Geometry check sheet. Reference: the model listing, model coordinates, mm. Face numbers are marked on the shaded views. A direction names the side the tool comes from. Give positions to 0.01 mm unless a question says otherwise; leave off trailing zeros. Write each loop counter-clockwise with the first axis right and the second up, starting at its lowest first coordinate (ties: lowest second). Pieces come first, ordered by that corner, then holes.
(1) Depth check by flat-ended pin: P1, Ø13, axis at x = 10, z = 35.5, coming from the -Y side; P2, Ø3, axis at y = 114.5, z = 40, coming from the -X side; P3, Ø12, axis at x = 17, y = 60.5, coming from the -Z side; P4, Ø13, axis at x = 16, z = 33.5, coming from the -Y side. Enter the tip coordinate at first touch or a pass-through.
(2) Thickness scan on line 1 along Z through (x, y) = (3, 41); line 2 along Y through (x, z) = (19, 22.86); line 3 along Z through (x, y) = (8.5, 0). Record the ranges inside material, lowest first.
(3) Cross-section at B-B (x = 12.7). Count the separate pieces of the cut face and the enclosed holes in it, and give its area (3 significant figures).
(4) Cross-section at A-A (y = 215.9). Record the boundary of the cut face in (x, z).
(5) Tool access check on the marked faces 5, 6 and 7. Record the directions out of +Z, -Z, +X, -X, +Y, -Y that give a thin tool (end or side, any length) a straight path to the whole face; none if there is none.
(6) Mould release check, pull along Z, two halves, no side actions. Record for the marked faces 1, 2, 3 and 4: +Z half, -Z half, draft (parallel to the pull), parting line (faces both ways), or undercut.
```python
from build123d import *

# Parameters (mm, degrees)
SKETCH3_W               = 50.8
SKETCH3_H               = 254
BOSS_EXTRUDE1_DEPTH     = 25.4
SKETCH4_R               = 4.7117
CUT_EXTRUDE1_DEPTH      = 246.225128402
SKETCH5_R               = 2.413
CUT_EXTRUDE2_DEPTH      = 246.225128402
SKETCH6_W               = 45.72
SKETCH6_H               = 85.725
CUT_EXTRUDE3_DEPTH      = 246.225128402
SKETCH7_W               = 15.24
SKETCH7_H               = 85.725
CUT_EXTRUDE4_DEPTH      = 1.4986
SKETCH8_W               = 15.24
SKETCH8_H               = 85.725
CUT_EXTRUDE5_DEPTH      = 1.4986
SKETCH9_W               = 30.48
SKETCH9_H               = 230.759
CUT_EXTRUDE6_DEPTH      = 246.225128402
FILLET5_R               = 6.35
SKETCH14_W              = 25.4
SKETCH14_H              = 254
BOSS_EXTRUDE2_DEPTH     = 12.7
FILLET8_R               = 38.1
FILLET9_R               = 9.525
FILLET10_R              = 10.16
FILLET11_R              = 15.24
FILLET12_R              = 5.08
SKETCH18_R              = 2.413
CUT_EXTRUDE8_DEPTH      = 251.804904258
CUT_EXTRUDE9_DEPTH      = 248.386090151
FILLET13_R              = 3.175
SKETCH20_R              = 6.35
CUT_EXTRUDE10_DEPTH     = 248.386090151
CUT_EXTRUDE11_START     = -254
CUT_EXTRUDE11_OUTLINE_W = 1.4986
CUT_EXTRUDE11_OUTLINE_H = 63.5
CUT_EXTRUDE11_DEPTH     = 254


# Read off the part's stored shape, not the designer's step: Cut-Extrude11
with BuildPart() as part:
    # Sketch3 → Boss-Extrude1 (new body)
    with BuildSketch(Plane(origin=(0, 0, 0), x_dir=(0, 0, -1), z_dir=(1, 0, 0))):
        with Locations((-10.16, 114.3)):
            Rectangle(SKETCH3_W, SKETCH3_H)
    extrude(amount=BOSS_EXTRUDE1_DEPTH)

    # Sketch4 → Cut-Extrude1 (cut, through all)
    with BuildSketch(Plane(origin=(0, 0, 0), x_dir=(0, 0, -1), z_dir=(1, 0, 0))):
        Circle(SKETCH4_R)
    extrude(amount=CUT_EXTRUDE1_DEPTH, mode=Mode.SUBTRACT)

    # Sketch5 → Cut-Extrude2 (cut, through all)
    with BuildSketch(Plane(origin=(0, 0, 0), x_dir=(0, 0, -1), z_dir=(1, 0, 0))):
        with Locations((-22.86, 70.866)):
            Circle(SKETCH5_R)
        with Locations((-22.86, 45.466)):
            Circle(SKETCH5_R)
    extrude(amount=CUT_EXTRUDE2_DEPTH, mode=Mode.SUBTRACT)

    # Sketch6 → Cut-Extrude3 (cut, through all)
    with BuildSketch(Plane(origin=(0, 0, 0), x_dir=(0, 0, -1), z_dir=(1, 0, 0))):
        with Locations((7.62, 53.4035)):
            Rectangle(SKETCH6_W, SKETCH6_H)
    extrude(amount=CUT_EXTRUDE3_DEPTH, mode=Mode.SUBTRACT)

    # Sketch7 → Cut-Extrude4 (cut)
    with BuildSketch(Plane(origin=(25.4, 0, 0), x_dir=(0, 0, -1), z_dir=(1, 0, 0))):
        with Locations((-22.86, 53.4035)):
            Rectangle(SKETCH7_W, SKETCH7_H)
    extrude(amount=-CUT_EXTRUDE4_DEPTH, mode=Mode.SUBTRACT)

    # Sketch8 → Cut-Extrude5 (cut)
    with BuildSketch(Plane.ZY):
        with Locations((22.86, 53.4035)):
            Rectangle(SKETCH8_W, SKETCH8_H)
    extrude(amount=-CUT_EXTRUDE5_DEPTH, mode=Mode.SUBTRACT)

    # Sketch9 → Cut-Extrude6 (cut, through all)
    with BuildSketch(Plane(origin=(25.4, 0, 0), x_dir=(0, 0, -1), z_dir=(1, 0, 0))):
        with Locations((0, 125.9205)):
            Rectangle(SKETCH9_W, SKETCH9_H)
    extrude(amount=-CUT_EXTRUDE6_DEPTH, mode=Mode.SUBTRACT)

    # Fillet5
    fillet5_edges = [part.edges().sort_by_distance(p)[0] for p in [
        (24.6507, 10.541, 30.48),
        (24.6507, 96.266, 30.48),
        (0.7493, 96.266, 30.48),
        (0.7493, 10.541, 30.48),
    ]]
    fillet(fillet5_edges, radius=FILLET5_R)

    # Sketch14 → Boss-Extrude2 (add)
    with BuildSketch(Plane.XY.offset(35.56)):
        with Locations((12.7, 114.3)):
            Rectangle(SKETCH14_W, SKETCH14_H)
    extrude(amount=BOSS_EXTRUDE2_DEPTH)

    # Fillet8
    fillet8_edges = [part.edges().sort_by_distance(p)[0] for p in [
        (12.7, -12.7, 48.26),
    ]]
    fillet(fillet8_edges, radius=FILLET8_R)

    # Fillet9
    fillet9_edges = [part.edges().sort_by_distance(p)[0] for p in [
        (12.7, 10.541, 15.24),
    ]]
    fillet(fillet9_edges, radius=FILLET9_R)

    # Fillet10
    fillet10_edges = [part.edges().sort_by_distance(p)[0] for p in [
        (12.7, 10.541, -15.24),
        (12.7, -12.7, -15.24),
    ]]
    fillet(fillet10_edges, radius=FILLET10_R)

    # Fillet11
    fillet11_edges = [part.edges().sort_by_distance(p)[0] for p in [
        (12.7, 241.3, 15.24),
    ]]
    fillet(fillet11_edges, radius=FILLET11_R)

    # Fillet12
    fillet12_edges = [part.edges().sort_by_distance(p)[0] for p in [
        (12.7, 241.3, 48.26),
    ]]
    fillet(fillet12_edges, radius=FILLET12_R)

    # Sketch18 → Cut-Extrude8 (cut, through all)
    with BuildSketch(Plane.XY.offset(48.26)):
        with Locations((12.7, 215.9)):
            Circle(SKETCH18_R)
        with Locations((12.7, 171.45)):
            Circle(SKETCH18_R)
    extrude(amount=-CUT_EXTRUDE8_DEPTH, mode=Mode.SUBTRACT)

    # Sketch19 → Cut-Extrude9 (cut, through all)
    with BuildSketch(Plane(origin=(25.4, 0, 0), x_dir=(0, 0, -1), z_dir=(1, 0, 0))):
        Polygon((-20.32, 110.399743879), (-43.18, 133.259743879), (-43.18, 110.399743879), (-43.18, 87.539743879), align=None)
        Polygon((-43.18, 137.749871939), (-20.32, 114.889871939), (-20.32, 160.609871939), align=None)
        Polygon((-43.18, 165.1), (-20.32, 165.1), (-43.18, 142.24), align=None)
        Polygon((-43.18, 206.375), (-20.32, 206.375), (-43.18, 183.515), align=None)
        Polygon((-43.18, 179.024871939), (-20.32, 201.884871939), (-20.32, 179.024871939), align=None)
    extrude(amount=-CUT_EXTRUDE9_DEPTH, mode=Mode.SUBTRACT)

    # Fillet13
    fillet13_edges = [part.edges().sort_by_distance(p)[0] for p in [
        (12.7, 87.539743879, 43.18),
        (12.7, 133.259743879, 43.18),
        (12.7, 110.399743879, 20.32),
        (12.7, 137.749871939, 43.18),
        (12.7, 160.609871939, 20.32),
        (12.7, 114.889871939, 20.32),
        (12.7, 142.24, 43.18),
        (12.7, 165.1, 43.18),
        (12.7, 165.1, 20.32),
        (12.7, 183.515, 43.18),
        (12.7, 206.375, 43.18),
        (12.7, 206.375, 20.32),
        (12.7, 179.024871939, 20.32),
        (12.7, 179.024871939, 43.18),
        (12.7, 201.884871939, 20.32),
    ]]
    fillet(fillet13_edges, radius=FILLET13_R)

    # Sketch20 → Cut-Extrude10 (cut, through all)
    with BuildSketch(Plane(origin=(25.4, 0, 0), x_dir=(0, 0, -1), z_dir=(1, 0, 0))):
        with Locations((-31.75, 228.6)):
            Circle(SKETCH20_R)
    extrude(amount=-CUT_EXTRUDE10_DEPTH, mode=Mode.SUBTRACT)

    # Cut-Extrude11 outline → Cut-Extrude11 (cut)
    with BuildSketch(Plane.XZ.offset(12.7).offset(CUT_EXTRUDE11_START)):
        with Locations((24.6507, 16.51)):
            Rectangle(CUT_EXTRUDE11_OUTLINE_W, CUT_EXTRUDE11_OUTLINE_H)
        with Locations((0.7493, 16.51)):
            Rectangle(CUT_EXTRUDE11_OUTLINE_W, CUT_EXTRUDE11_OUTLINE_H)
    extrude(amount=CUT_EXTRUDE11_DEPTH, mode=Mode.SUBTRACT)


solid = part.part
```
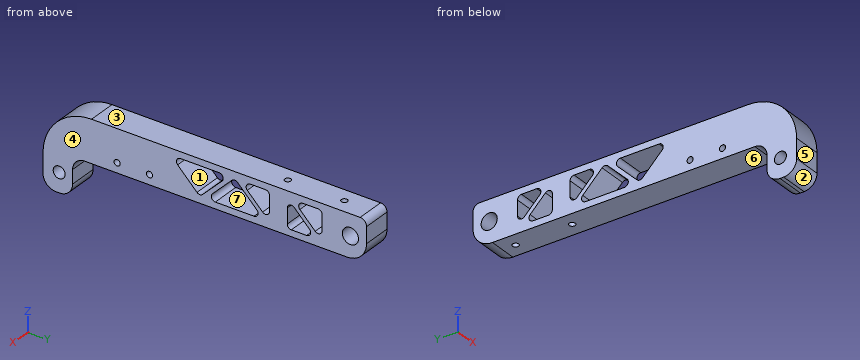
Reply:
1. P1: stops at y = -7.72
1. P2: passes through
1. P3: stops at z = 15.24
1. P4: stops at y = -8.78
2. line 1: z = 15.24 to 48.26
2. line 2: y = -10.52 to 43.05, 47.88 to 68.45, 73.28 to 107.86, 112.94 to 119.44, 156.06 to 179.09, 197.33 to 239.26
2. line 3: z = -15.24 to -4.71, 4.71 to 38.56
3. separate pieces: 3
3. enclosed holes: 9
3. area: 6,460 mm2
4. outline: (1.5, 15.24) - (10.29, 15.24) - (10.29, 48.26) - (1.5, 48.26) - close; (15.11, 15.24) - (23.9, 15.24) - (23.9, 48.26) - (15.11, 48.26) - close
5. face 5: +Z, -Z, +X, -X, -Y
5. face 6: -Z, +X, -X, +Y
5. face 7: +X, -X
6. face 1: undercut
6. face 2: -Z half
6. face 3: +Z half
6. face 4: draft
